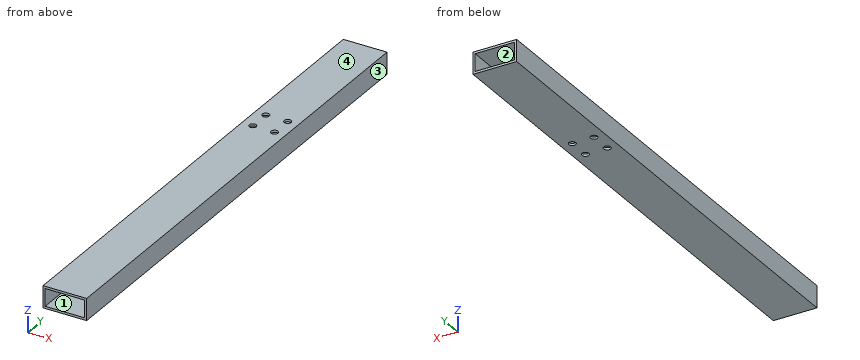
from build123d import *

# Parameters (mm, degrees)
SKETCH_1_W          = 20
SKETCH_1_H          = 10
SKETCH_1_W_2        = 18
SKETCH_1_H_2        = 8
EXTRUDE_1_DEPTH     = 230
SKETCH_3_R          = 1.6
CUT_EXTRUDE_1_DEPTH = 231.434372436


with BuildPart() as part:
    # 草图1 → 拉伸-薄壁1 (new body)
    with BuildSketch(Plane(origin=(0, 0, 0), x_dir=(1, 0, 0), z_dir=(0, 1, 0))):
        Rectangle(SKETCH_1_W, SKETCH_1_H)
        Rectangle(SKETCH_1_W_2, SKETCH_1_H_2, mode=Mode.SUBTRACT)
    extrude(amount=EXTRUDE_1_DEPTH)

    # 草图3 → 切除-拉伸1 (cut, through all)
    with BuildSketch(Plane.XY.offset(5)):
        with Locations((-5, 162.3)):
            Circle(SKETCH_3_R)
        with Locations(Location((-5, 152.3, 0), (0, 0, 180))):
            Circle(SKETCH_3_R)
        with Locations((5, 152.3)):
            Circle(SKETCH_3_R)
        with Locations(Location((5, 162.3, 0), (0, 0, 180))):
            Circle(SKETCH_3_R)
    extrude(amount=-CUT_EXTRUDE_1_DEPTH, mode=Mode.SUBTRACT)


solid = part.part
Could you check a few things on this model? Use its own coordinates, in mm. Face numbers are marked on the shaded views. Give positions to 0.01 mm unless a question says otherwise; leave off trailing zeros. Order: outer loops, then holes, each group sorted by start corner. A loop starts at its lowest first (then second) coordinate and runs counter-clockwise, first axis right, second up.
1. Suppose I cut it at B-B (z = 0). List the corners of the cut face in (x, y) for me.
2. We'd pull the mould along Z, two halves only. Please class the marked faces 1, 2, 3 and 4: pulls with the +Z half, pulls with the -Z half, needs draft (parallel to the pull), parting line crosses it, or undercut.
3. Suppose I cut it at A-A (x = -0.75). List the corners of the cut face in (y, z) for me, plus the area to 3 significant figures.
4. I need wall thicknesses on L1, parallel to Y at x = 5, z = -4.55; L2, parallel to X at y = 162.3, z = 4.7; L3, parallel to Z at x = 2.75, y = 128. Which ranges of each line are inside material? Lowest first, please.
5. Will this pin go through, and if not, where does the flat tip stop? P1, Ø3, axis at x = -5, y = 152.3, coming from the +Z side.
6. Suppose I cut it at C-C (y = 50). List the corners of the cut face in (x, z) for me, plus the area to 3 significant figures.
Solved:
1. outline: (-10, 0) - (-9, 0) - (-9, 230) - (-10, 230) - close; (9, 0) - (10, 0) - (10, 230) - (9, 230) - close
2. face 1: undercut
2. face 2: undercut
2. face 3: needs draft
2. face 4: pulls with the +Z half
3. outline: (0, -5) - (230, -5) - (230, -4) - (0, -4) - close; (0, 4) - (230, 4) - (230, 5) - (0, 5) - close
3. area: 460 mm2
4. L1: y = 0 to 150.7, 153.9 to 160.7, 163.9 to 230
4. L2: x = -10 to -6.6, -3.4 to 3.4, 6.6 to 10
4. L3: z = -5 to -4, 4 to 5
5. P1: passes through
6. outline: (-10, -5) - (10, -5) - (10, 5) - (-10, 5) - close; hole (-9, -4) - (9, -4) - (9, 4) - (-9, 4) - close
6. area: 56.0 mm2
